Here's how the part is built. I have some questions about the finished solid (model axes, mm). Face numbers are marked on the shaded views. Coordinates: 2 decimals unless noted, no trailing zeros. Loops run counter-clockwise (first coordinate to the right, second up) from the corner with the lowest first, then second, coordinate; pieces in that order, holes last. Notation, with made-up numbers: (15, 43.5) -> (42, 43.5) arc R36 ccw to (42, 78.5) -> close; hole circle Ø9 at (52.5, -28.5). An arc over 180 degrees is marked (long way). Answer as a JSON object with one key per item and string values. Group by question number.
Q1. I want a section at C-C on y = -4. Write out the boundary of the cut face in (x, z), then the cut area to 3 significant figures.
Q2. I want a section at B-B on z = -6.25. Write out the boundary of the cut face in (x, y).
Q3. I want a section at A-A on x = 3.65. Write out the boundary of the cut face in (y, z).
Q4. I need wall thicknesses on line 1 (Z direction, x = 3.65, y = -2.25); line 2 (X direction, y = -5.75, z = 6.5); line 3 (Z direction, x = 4.75, y = -2.75). Which ranges of each line are inside material? Lowest first, please.
Q5. Thinking about a two-plate mould opening in Z: for the marked faces 1, 2 and 3, which applies, released by +Z, released by -Z, zero draft, split by the parting line, or undercut?
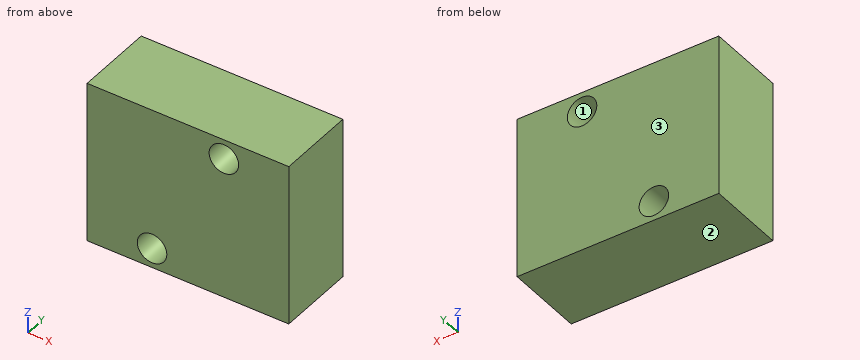
```python
from build123d import *

# Parameters (mm, degrees)
F0_W     = 20.5
F0_H     = 16.5
F1_DEPTH = 8
F2_R     = 1.5
F3_DEPTH = 25
F4_DEPTH = 25
F5_DEPTH = 25


with BuildPart() as f1:
    # F0 (on Front) → F1 (new body)
    with BuildSketch(Plane.XZ):
        Rectangle(F0_W, F0_H)
    extrude(amount=F1_DEPTH)

    # F2 (on face) → F3 (cut)
    with BuildSketch(Plane.XZ.offset(8)):
        with Locations((3.65, 6.25)):
            Circle(F2_R)
        with Locations((-3.65, -6.25)):
            Circle(F2_R)
    extrude(amount=-F3_DEPTH, mode=Mode.SUBTRACT)

    # F2 (on face) → F4 (cut)
    with BuildSketch(Plane.XZ.offset(8)):
        with Locations((3.65, 6.25)):
            Circle(F2_R)
        with Locations((-3.65, -6.25)):
            Circle(F2_R)
    extrude(amount=-F4_DEPTH, mode=Mode.SUBTRACT)

    # F2 (on face) → F5 (cut)
    with BuildSketch(Plane.XZ.offset(8)):
        with Locations((3.65, 6.25)):
            Circle(F2_R)
        with Locations((-3.65, -6.25)):
            Circle(F2_R)
    extrude(amount=-F5_DEPTH, mode=Mode.SUBTRACT)


solid = f1.part
```
Result set:
{
 "1": {"outline": "(-10.25, -8.25) -> (10.25, -8.25) -> (10.25, 8.25) -> (-10.25, 8.25) -> close; hole circle Ø3 at (-3.65, -6.25); hole circle Ø3 at (3.65, 6.25)", "area": "324 mm²"},
 "2": {"outline": "(-10.25, -8) -> (-5.15, -8) -> (-5.15, 0) -> (-10.25, 0) -> close; (-2.15, -8) -> (10.25, -8) -> (10.25, 0) -> (-2.15, 0) -> close"},
 "3": {"outline": "(-8, -8.25) -> (0, -8.25) -> (0, 4.75) -> (-8, 4.75) -> close; (-8, 7.75) -> (0, 7.75) -> (0, 8.25) -> (-8, 8.25) -> close"},
 "4": {"line 1": "z = -8.25 to 4.75, 7.75 to 8.25", "line 2": "x = -10.25 to 2.17, 5.13 to 10.25", "line 3": "z = -8.25 to 5.23, 7.27 to 8.25"},
 "5": {"face 1": "undercut", "face 2": "released by -Z", "face 3": "zero draft"}
}
